from build123d import *

# Parameters (mm, degrees)
SKETCH_1_W          = 200
SKETCH_1_H          = 200
EXTRUDE_1_DEPTH     = 200
CHAMFER_1_SIZE      = 18
SKETCH_2_R          = 57.5
CUT_EXTRUDE_1_DEPTH = 150
SKETCH_3_R          = 52.5
SKETCH_3_R_2        = 50
CUT_EXTRUDE_4_DEPTH = 5


with BuildPart() as part:
    # Sketch 1 → Extrude 1 (new body)
    with BuildSketch(Plane(origin=(0, 0, 0), x_dir=(0, 0, -1), z_dir=(1, 0, 0))):
        with Locations((100, 100)):
            Rectangle(SKETCH_1_W, SKETCH_1_H)
    extrude(amount=EXTRUDE_1_DEPTH)

    # Chamfer 1
    chamfer_1_edges = [part.edges().sort_by_distance(p)[0] for p in [
        (200, 100, -200),
        (200, 200, -100),
        (200, 100, 0),
        (0, 200, -100),
        (0, 100, -200),
        (0, 0, -100),
        (0, 100, 0),
        (200, 0, -100),
        (100, 200, 0),
        (100, 200, -200),
        (100, 0, -200),
        (100, 0, 0),
    ]]
    chamfer(chamfer_1_edges, length=CHAMFER_1_SIZE)

    # Sketch 2 → Cut-Extrude 1 (cut)
    with BuildSketch(Plane(origin=(0, 200, 0), x_dir=(1, 0, 0), z_dir=(0, 1, 0))):
        with Locations(Location((100, 100, 0), (0, 0, 270))):
            Circle(SKETCH_2_R)
    extrude(amount=-CUT_EXTRUDE_1_DEPTH, mode=Mode.SUBTRACT)

    # Sketch 3 → Cut-Extrude 4 (cut)
    with BuildSketch(Plane.XY):
        with Locations((100, 100)):
            Circle(SKETCH_3_R)
        with Locations((100, 100)):
            Circle(SKETCH_3_R_2, mode=Mode.SUBTRACT)
        with BuildLine():
            add(Edge.make_bspline(
                [(124.952810184, 122.311754672), (124.061928668, 122.316141415), (122.723328375, 122.065314477), (121.15976707, 121.17726781), (120.31812048, 120.404799304), (119.711791362, 119.661639483), (119.299662129, 118.992437635), (118.890623993, 118.246055909), (118.558018296, 117.387310251), (118.225423141, 116.448647339), (117.836741696, 115.008969129), (117.587459376, 113.876131637), (117.476848645, 113.080985442)],
                knots=[0, 0, 0, 0, 0.204127863, 0.304431221, 0.408409421, 0.463887314, 0.523727039, 0.588196002, 0.658593566, 0.734357814, 0.816313439, 1, 1, 1, 1], degree=3))
            Line((117.476848645, 113.080985442), (106.707617876, 113.080985442))
            add(Edge.make_bspline(
                [(106.707617876, 113.080985442), (106.781895264, 114.937649447), (107.131475338, 117.664732571), (108.237782966, 121.070374863), (109.302543269, 123.370468484), (110.613437766, 125.442055382), (112.132515124, 127.267990733), (113.875631172, 128.806059043), (115.795871388, 130.092952145), (117.895783577, 131.088301864), (120.9374414, 132.05768373), (123.358242769, 132.306151558), (124.988867876, 132.311754672)],
                knots=[0, 0, 0, 0, 0.188116369, 0.27589316, 0.361277617, 0.44378986, 0.523169186, 0.600666658, 0.678099482, 0.756216315, 0.834899655, 1, 1, 1, 1], degree=3))
            add(Edge.make_bspline(
                [(124.988867876, 132.311754672), (126.175754308, 132.315676764), (127.93496111, 132.179510664), (130.186678669, 131.655134145), (131.7726869, 131.129273666), (133.268472003, 130.437845008), (134.687294958, 129.602483287), (136.026293603, 128.613446176), (137.265267034, 127.476325352), (138.390653811, 126.231694174), (139.384787852, 124.902245602), (140.228434325, 123.499377361), (140.906924261, 122.013604885), (141.434573231, 120.458552141), (141.959304994, 118.255123496), (142.09551179, 116.535641705), (142.092233261, 115.376658519)],
                knots=[0, 0, 0, 0, 0.132319326, 0.195567087, 0.25726574, 0.318197153, 0.378841636, 0.440456231, 0.50334526, 0.56593404, 0.627190101, 0.688062599, 0.747996218, 0.808849065, 0.870792773, 1, 1, 1, 1], degree=3))
            add(Edge.make_bspline(
                [(142.092233261, 115.376658519), (142.09732202, 114.393518355), (141.95430932, 112.905639606), (141.581070463, 110.915109319), (141.148217608, 109.37826343), (140.624528159, 107.801834253), (139.967531924, 106.199142481), (139.199146108, 104.565449003), (138.455218348, 103.183260504), (137.779650529, 102.028028639), (137.171822841, 101.090201616), (136.490804976, 100.08130842), (135.711268931, 99.01064295), (134.866860384, 97.854812526), (133.910144174, 96.645058775), (132.880240035, 95.363192003), (131.771215601, 94.008863585), (130.567357552, 92.595436285), (129.285008389, 91.105753441), (127.911135514, 89.550736384), (126.443361597, 87.93660771), (124.906447454, 86.233134327), (122.679244122, 83.836732523), (120.967131822, 82.003308094), (119.784540953, 80.773293134)],
                knots=[0, 0, 0, 0, 0.069981715, 0.106336674, 0.144238498, 0.183709243, 0.224708791, 0.267639701, 0.312364973, 0.33656381, 0.36302672, 0.392021296, 0.423331852, 0.457435971, 0.494060334, 0.533269791, 0.574668339, 0.618846706, 0.665626965, 0.714798059, 0.766769623, 0.82116182, 0.878361292, 1, 1, 1, 1], degree=3))
            Line((119.784540953, 80.773293134), (139.784540953, 80.773293134))
            Line((139.784540953, 80.773293134), (138.462425568, 70.773293134))
            Line((138.462425568, 70.773293134), (102.092233261, 70.773293134))
            Line((102.092233261, 70.773293134), (102.86146403, 78.465600826))
            add(Edge.make_bspline(
                [(102.86146403, 78.465600826), (104.073053727, 79.737856076), (105.861414534, 81.588001167), (108.15811719, 84.030126363), (109.77444844, 85.719605027), (111.292181295, 87.342421418), (112.742192845, 88.873377879), (114.109044196, 90.319346392), (115.381760254, 91.694514713), (116.578546994, 92.97827206), (117.673765861, 94.197556125), (118.717301158, 95.306997342), (119.650706014, 96.356133448), (120.503599196, 97.32161107), (121.495876039, 98.422484298), (122.172586535, 99.230130727), (122.609060184, 99.727620057)],
                knots=[0, 0, 0, 0, 0.181614482, 0.265988361, 0.346548719, 0.423311675, 0.495675135, 0.564525855, 0.628995855, 0.68936882, 0.745950656, 0.798411213, 0.846803604, 0.891102717, 0.931584129, 1, 1, 1, 1], degree=3))
            add(Edge.make_bspline(
                [(122.609060184, 99.727620057), (123.542457488, 100.855288981), (124.884611957, 102.474543208), (126.494767665, 104.618871476), (127.522861077, 106.015472175), (128.390657407, 107.310563545), (129.306154563, 108.764488546), (129.869005007, 109.828049592), (130.157137107, 110.508870057)],
                knots=[0, 0, 0, 0, 0.332831745, 0.477817127, 0.609520417, 0.726973213, 0.832099586, 1, 1, 1, 1], degree=3))
            add(Edge.make_bspline(
                [(130.157137107, 110.508870057), (130.511822539, 111.366072382), (131.120426847, 113.057426489), (131.319730922, 114.845166367), (131.323002492, 115.701177749)],
                knots=[0, 0, 0, 0, 0.520562004, 1, 1, 1, 1], degree=3))
            add(Edge.make_bspline(
                [(131.323002492, 115.701177749), (131.302782595, 116.579231828), (131.136297941, 117.914660904), (130.3064802, 119.455009614), (129.500708922, 120.45075585), (128.538845138, 121.277303266), (127.061812678, 122.101056155), (125.792809521, 122.304509149), (124.952810184, 122.311754672)],
                knots=[0, 0, 0, 0, 0.259693846, 0.38313667, 0.508398189, 0.633351073, 0.752658268, 1, 1, 1, 1], degree=3))
        make_face()
        Polygon((55.169156338, 91.951177749), (87.140310184, 132.311754672), (97.585021722, 132.311754672), (91.960021722, 91.542523903), (97.837425568, 91.542523903), (96.539348645, 81.542523903), (90.589829415, 81.542523903), (89.099444799, 70.773293134), (78.246079415, 70.773293134), (79.73646403, 81.542523903), (54.399925568, 81.542523903), align=None)
        Polygon((81.106656338, 91.542523903), (84.207617876, 114.018485442), (66.407137107, 91.542523903), align=None, mode=Mode.SUBTRACT)
    extrude(amount=-CUT_EXTRUDE_4_DEPTH, mode=Mode.SUBTRACT)


solid = part.part
CAD build for the part. Positions are in the model's coordinates, mm. A direction names the side the tool comes from. Round coordinates to 2 decimals unless told otherwise and drop trailing zeros. Write each loop counter-clockwise with the first axis right and the second up, starting at its lowest first coordinate (ties: lowest second). Pieces come first, ordered by that corner, then holes. Notation, with made-up numbers: M -29,-2.5 L -5,-2.5 A22 ccw -5,25.5 Z; hole C -12,84.25 d7. An arc over 180 degrees is marked long. Use a Markdown table: item, result. Add a question column.
1. Drill centre lines: probe 1 along Y at (x, z) = (100, -3.5); probe 2 along Y at (x, z) = (100, -2); probe 3 along X at (y, z) = (101, -100). Where is each one in solid material? Low to high.
2. Flat gauge pins, fed straight in: P1, Ø2.5, axis at x = 85, z = -3, coming from the +Y side; P2, Ø5.5, axis at x = 94.5, z = -2.5, coming from the -Y side; P3, Ø2.5, axis at x = 92.5, z = -2, coming from the +Y side; P4, Ø13, axis at x = 72.5, y = 107.5, coming from the +Z side. Where does each tip first touch, or does it go through?
3. 3-axis set-ups, long thin cutter, end or side, ignore diameter. For faces 5 (the face through (62, 62, 0)), 6 (the face through (127, 102, -5)): which of +Z, -Z, +X, -X, +Y, -Y reach the whole face in a straight line?
4. Slice it at B-B on x = 174.5. Give the cut face in (y, z), then the cut area to 3 significant figures.
5. Slice it at D-D on z = -100. Give the cut face in (x, y).
6. Slice it at A-A on z = -185.5. Give the cut face in (x, y).
7. Pull direction X, two halves, no side cores. Call faces 1 (the face through (138.86, 126.05, -142.38)), 2 (the face through (99, 0, -99)), 3 (the face through (70.93, 111.85, -2.46)), 4 (the face through (12, 11, -187)): released by +X, released by -X, zero draft, split by the parting line, or undercut.
8. Slice it at C-C on y = 58. Give the cut face in (x, z).
Reply:
| question | item | result |
|---|---|---|
| 1 | probe 1 | y = 14.5 to 47.5, 50 to 150, 152.5 to 185.5 |
| 1 | probe 2 | y = 16 to 47.5, 50 to 150, 152.5 to 184 |
| 1 | probe 3 | x = 0 to 42.5, 157.5 to 200 |
| 2 | P1 | stops at y = 186.25 |
| 2 | P2 | stops at y = 12.75 |
| 2 | P3 | stops at y = 185.25 |
| 2 | P4 | stops at z = 0 |
| 3 | face 5 | +Z, +X, -X, +Y, -Y |
| 3 | face 6 | +Z |
| 4 | outline | M 0,-182 L 18,-200 L 182,-200 L 200,-182 L 200,-18 L 182,0 L 18,0 L 0,-18 Z |
| 4 | area | 39,400 mm^2 |
| 5 | outline | M 0,18 L 18,0 L 182,0 L 200,18 L 200,182 L 182,200 L 157.5,200 L 157.5,50 L 42.5,50 L 42.5,200 L 18,200 L 0,182 Z |
| 6 | outline | M 3.5,18 L 18,3.5 L 182,3.5 L 196.5,18 L 196.5,182 L 182,196.5 L 18,196.5 L 3.5,182 Z |
| 7 | face 1 | undercut |
| 7 | face 2 | zero draft |
| 7 | face 3 | undercut |
| 7 | face 4 | released by -X |
| 8 | outline | M 0,-182 L 18,-200 L 182,-200 L 200,-182 L 200,-18 L 182,0 L 131.5,0 L 131.5,-5 L 127.13,-5 L 127.13,0 L 72.87,0 L 72.87,-5 L 68.5,-5 L 68.5,0 L 18,0 L 0,-18 Z; hole C 100,-100 d115 |
